Geometry: final body of the model. Coordinates: model frame, mm. A direction names the side the tool comes from. Coordinates: 2 decimals unless noted, no trailing zeros. Order: outer loops, then holes, each group sorted by start corner. A loop starts at its lowest first (then second) coordinate and runs counter-clockwise, first axis right, second up. Notation, with made-up numbers: M 86,73.5 L 114,73.5 A16 ccw 114,77.5 Z; hole C 77,40 d7. An arc over 180 degrees is marked long. One line per question, with ' | ' between items.
from build123d import *

# Parameters (mm, degrees)
SKETCH_W        = 100
SKETCH_H        = 84
PAD_DEPTH       = 10
SKETCH001_R     = 2.1
POCKET_DEPTH    = 10
SKETCH002_R     = 2.1
POCKET001_DEPTH = 10
SKETCH003_R     = 4
POCKET002_DEPTH = 4
SKETCH004_R     = 4
POCKET003_DEPTH = 4
SKETCH005_R     = 3.1
POCKET004_DEPTH = 10
SKETCH006_R     = 4.8
POCKET005_DEPTH = 5.2
FILLET_R        = 2


with BuildPart() as part:
    # Sketch → Pad (new body)
    with BuildSketch(Plane.XY):
        with Locations((50, 42)):
            Rectangle(SKETCH_W, SKETCH_H)
    extrude(amount=PAD_DEPTH)

    # Sketch001 (on Face6 of Pad) → Pocket (cut)
    with BuildSketch(Plane.XY.offset(10)):
        with Locations((5, 6)):
            Circle(SKETCH001_R)
        with Locations((29, 6)):
            Circle(SKETCH001_R)
        with Locations((71, 6)):
            Circle(SKETCH001_R)
        with Locations((95, 6)):
            Circle(SKETCH001_R)
        with Locations((5, 24)):
            Circle(SKETCH001_R)
        with Locations((29, 24)):
            Circle(SKETCH001_R)
        with Locations((71, 24)):
            Circle(SKETCH001_R)
        with Locations((95, 24)):
            Circle(SKETCH001_R)
        with Locations((5, 78)):
            Circle(SKETCH001_R)
        with Locations((29, 78)):
            Circle(SKETCH001_R)
        with Locations((5, 60)):
            Circle(SKETCH001_R)
        with Locations((29, 60)):
            Circle(SKETCH001_R)
        with Locations((71, 78)):
            Circle(SKETCH001_R)
        with Locations((95, 78)):
            Circle(SKETCH001_R)
        with Locations((71, 60)):
            Circle(SKETCH001_R)
        with Locations((95, 60)):
            Circle(SKETCH001_R)
    extrude(amount=-POCKET_DEPTH, mode=Mode.SUBTRACT)

    # Sketch002 (on Face5 of Pocket) → Pocket001 (cut)
    with BuildSketch(Plane.XY.offset(10)):
        with Locations((35, 47)):
            Circle(SKETCH002_R)
        with Locations((65, 47)):
            Circle(SKETCH002_R)
        with Locations((35, 37)):
            Circle(SKETCH002_R)
        with Locations((65, 37)):
            Circle(SKETCH002_R)
    extrude(amount=-POCKET001_DEPTH, mode=Mode.SUBTRACT)

    # Sketch003 (on Face5 of Pocket001) → Pocket002 (cut)
    with BuildSketch(Plane.XY.offset(10)):
        with Locations((35, 47)):
            Circle(SKETCH003_R)
        with Locations((65, 47)):
            Circle(SKETCH003_R)
        with Locations((35, 37)):
            Circle(SKETCH003_R)
        with Locations((65, 37)):
            Circle(SKETCH003_R)
    extrude(amount=-POCKET002_DEPTH, mode=Mode.SUBTRACT)

    # Sketch004 (on Face5 of Pocket002) → Pocket003 (cut)
    with BuildSketch(Plane.XY.offset(10)):
        with Locations((5, 78)):
            Circle(SKETCH004_R)
        with Locations((29, 78)):
            Circle(SKETCH004_R)
        with Locations((5, 60)):
            Circle(SKETCH004_R)
        with Locations((29, 60)):
            Circle(SKETCH004_R)
        with Locations((5, 24)):
            Circle(SKETCH004_R)
        with Locations((29, 24)):
            Circle(SKETCH004_R)
        with Locations((5, 6)):
            Circle(SKETCH004_R)
        with Locations((29, 6)):
            Circle(SKETCH004_R)
        with Locations((71, 78)):
            Circle(SKETCH004_R)
        with Locations((71, 60)):
            Circle(SKETCH004_R)
        with Locations((95, 78)):
            Circle(SKETCH004_R)
        with Locations((95, 60)):
            Circle(SKETCH004_R)
        with Locations((71, 24)):
            Circle(SKETCH004_R)
        with Locations((95, 24)):
            Circle(SKETCH004_R)
        with Locations((71, 6)):
            Circle(SKETCH004_R)
        with Locations((95, 6)):
            Circle(SKETCH004_R)
    extrude(amount=-POCKET003_DEPTH, mode=Mode.SUBTRACT)

    # Sketch005 (on Face5 of Pocket003) → Pocket004 (cut)
    with BuildSketch(Plane.XY.offset(10)):
        with Locations((20, 62)):
            Circle(SKETCH005_R)
        with Locations((80, 62)):
            Circle(SKETCH005_R)
        with Locations((20, 22)):
            Circle(SKETCH005_R)
        with Locations((80, 22)):
            Circle(SKETCH005_R)
    extrude(amount=-POCKET004_DEPTH, mode=Mode.SUBTRACT)

    # Sketch006 (on Face4 of Pocket004) → Pocket005 (cut)
    with BuildSketch(Plane(origin=(0, 0, 0), x_dir=(1, 0, 0), z_dir=(0, 0, -1))):
        with Locations((20, -22)):
            Circle(SKETCH006_R)
        with Locations((20, -62)):
            Circle(SKETCH006_R)
        with Locations((80, -62)):
            Circle(SKETCH006_R)
        with Locations((80, -22)):
            Circle(SKETCH006_R)
    extrude(amount=-POCKET005_DEPTH, mode=Mode.SUBTRACT)

    # Fillet
    fillet_edges = [part.edges().sort_by_distance(p)[0] for p in [
        (0, 84, 5),
        (100, 84, 5),
        (0, 0, 5),
        (100, 0, 5),
    ]]
    fillet(fillet_edges, radius=FILLET_R)


solid = part.part
1. Section C-C, the plane z = 8.5. Give the number of separate pieces and of enclosed holes in the cut face, and give its area (3 significant figures).
Response values:
separate pieces: 1 | enclosed holes: 24 | area: 7,270 mm^2
2. Pin query (flat end, axial travel): P1, Ø6.5, axis at x = 29, y = 78, coming from the -Z side; P2, Ø4, axis at x = 30.5, y = 60.5, coming from the +Z side; P3, Ø2.5, axis at x = 5.5, y = 78, coming from the +Z side. Return the tip coordinate at first contact, or that it passes through.
Response values:
P1: stops at z = 0 | P2: stops at z = 6 | P3: passes through
3. Section A-A, the plane y = 37. Output: boundary loops of the cut face in (x, z).
Response values:
outline: M 0,0 L 32.9,0 L 32.9,6 L 31,6 L 31,10 L 0,10 Z; M 37.1,0 L 62.9,0 L 62.9,6 L 61,6 L 61,10 L 39,10 L 39,6 L 37.1,6 Z; M 67.1,0 L 100,0 L 100,10 L 69,10 L 69,6 L 67.1,6 Z
4. Section B-B, the plane x = 80. Output: boundary loops of the cut face in (y, z).
Response values:
outline: M 0,0 L 17.2,0 L 17.2,5.2 L 18.9,5.2 L 18.9,10 L 0,10 Z; M 25.1,5.2 L 26.8,5.2 L 26.8,0 L 57.2,0 L 57.2,5.2 L 58.9,5.2 L 58.9,10 L 25.1,10 Z; M 65.1,5.2 L 66.8,5.2 L 66.8,0 L 84,0 L 84,10 L 65.1,10 Z
5. Material intervals for line 1 (Y direction, x = 95, z = 1.9); line 2 (Y direction, x = 35, z = 8.2); line 3 (Y direction, x = 20, z = 3.5), sorted ascending. Write a range as [from, to].
Response values:
line 1: y = [0, 3.9], [8.1, 21.9], [26.1, 57.9], [62.1, 75.9], [80.1, 84] | line 2: y = [0, 33], [41, 43], [51, 84] | line 3: y = [0, 17.2], [26.8, 57.2], [66.8, 84]
6. Access query for faces 1 (the face through (81, 65.1, 5.2)), 2 (the face through (92.9, 6.09, 3.04)), 3 (the face through (31, 58, 6)). Directions: +Z, -Z, +X, -X, +Y, -Y. A direction counts if a zero-diameter tool reaches every point of the face in a straight line with its end or side. Return the directions, or none.
Response values:
face 1: -Z | face 2: +Z, -Z | face 3: +Z
